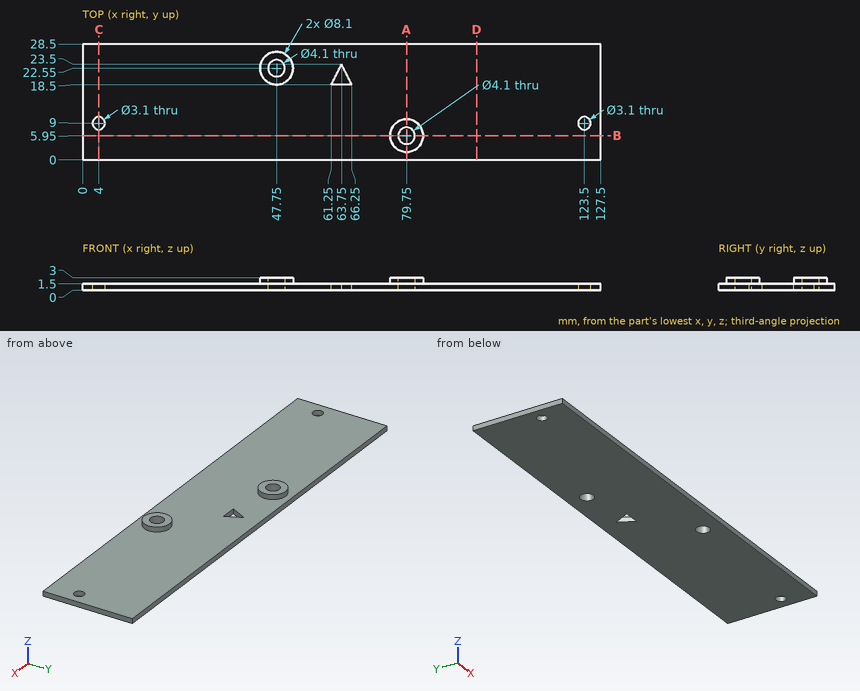
Input: dimensioned drawing with shaded views. Units: mm. Origin: part minimum x, y, z. Give positions to 0.01 mm unless a question says otherwise; leave off trailing zeros. Loops run counter-clockwise (first coordinate to the right, second up) from the corner with the lowest first, then second, coordinate; pieces in that order, holes last. Notation, with made-up numbers: M -25,80 L 13,80 A13 cw 13,97 Z; hole C 31.25,56.5 d5. An arc over 180 degrees is marked long. Put each result on its own line as item: value.
1) Material intervals for L1, parallel to Y at x = 123.5, z = 0.95; L2, parallel to Y at x = 47.75, z = 1.65; L3, parallel to X at y = 10.25, z = 0.7, sorted ascending. Write a range as from..to.
Computed values:
L1: y = 0..7.45, 10.55..28.5
L2: y = 18.5..20.5, 24.6..26.6
L3: x = 0..3.08, 4.92..122.58, 124.42..127.5
2) Cut plane D-D, the plane x = 97. Return the cut outline in (y, z), plus the area to 4 significant figures.
Computed values:
outline: M 0,0 L 28.5,0 L 28.5,1.5 L 0,1.5 Z
area: 42.75 mm^2
3) Cut plane B-B, the plane y = 5.95. Return the cut outline in (x, z).
Computed values:
outline: M 0,0 L 77.7,0 L 77.7,3 L 75.7,3 L 75.7,1.5 L 0,1.5 Z; M 81.8,0 L 127.5,0 L 127.5,1.5 L 83.8,1.5 L 83.8,3 L 81.8,3 Z
4) First-contact query: P1, Ø4, axis at x = 123.5, y = 9, coming from the +Z side; P2, Ø2.5, axis at x = 79.75, y = 5.95, coming from the -Z side. Flat tips, straight axial feed; report the tip coordinate or a pass-through.
Computed values:
P1: stops at z = 1.5
P2: passes through
5) Cut plane A-A, the plane x = 79.75. Return the cut outline in (y, z).
Computed values:
outline: M 0,0 L 3.9,0 L 3.9,3 L 1.9,3 L 1.9,1.5 L 0,1.5 Z; M 8,0 L 28.5,0 L 28.5,1.5 L 10,1.5 L 10,3 L 8,3 Z
6) Cut plane C-C, the plane x = 4. Return the cut outline in (y, z), plus the area to 3 significant figures.
Computed values:
outline: M 0,0 L 7.45,0 L 7.45,1.5 L 0,1.5 Z; M 10.55,0 L 28.5,0 L 28.5,1.5 L 10.55,1.5 Z
area: 38.1 mm^2
